Read the model definition and answer for the solid it produces. Units are mm, in the model's axes. A direction names the side the tool comes from. Give positions to 0.01 mm unless a question says otherwise; leave off trailing zeros. Loops run counter-clockwise (first coordinate to the right, second up) from the corner with the lowest first, then second, coordinate; pieces in that order, holes last. Notation, with made-up numbers: (67.25, 82) - (73.25, 82) arc R35 ccw to (73.25, 119) - close; hole circle Ø11 at (-22, 11). An arc over 180 degrees is marked (long way). Put each result on its own line as item: value. Start each with the question number.
1. A cutting plane is placed at A-A, the plane y = 29.5. Determine the outline of the cut face in (x, z), plus the area to 3 significant figures.
2. A cutting plane is placed at D-D, the plane z = 25. Determine the outline of the cut face in (x, y), plus the area to 3 significant figures.
3. For faces 1 (the flat face through (48.877, 46, 20)), 2 (the flat face through (-41.094, 22, 18)), determine the directions among +Z, -Z, +X, -X, +Y, -Y from which every point of the face is accessible in a straight line to the end or side of a thin tool.
4. Consider L1, parallel to X at y = 31, z = 15; L2, parallel to Y at x = 22, z = 8.5; L3, parallel to X at y = 91.5, z = 5. Determine where each line is inside the solid, lowest interval first. Write a range as from..to.
5. A cutting plane is placed at B-B, the plane z = 12. Determine the outline of the cut face in (x, y).
6. A cutting plane is placed at C-C, the plane x = -28. Determine the outline of the cut face in (y, z).
7. Given pin 1 Ø1.5 at (x, y) = (36, -1.5) entering from +Z; pin 2 Ø1.5 at (y, z) = (56.5, 32.5) entering from -X; pin 3 Ø12 at (x, z) = (16.5, 12.5) entering from +Y, each flat-ended and moving along its own axis, determine where each tip first touches the part or whether it passes through.
```python
from build123d import *

# Parameters (mm, degrees)
F0_W     = 11.016868
F0_H     = 24.481927
F0_W_2   = 8.267472
F0_H_2   = 10.750423
F0_W_3   = 4.593041
F0_W_4   = 12.248872
F0_W_5   = 4.59304
F1_DEPTH = 1.836145
F3_DEPTH = 44.06747
F5_DEPTH = 50.8


with BuildPart() as f1:
    # F0 (on Front) → F1 (new body)
    with BuildSketch(Plane.XZ):
        Polygon((-42.930589, 34.886747), (-42.930589, 0), (48.876639, 0), (48.876639, 38.559036), align=None)
        with Locations((-9.046323, 14.077108)):
            Rectangle(F0_W, F0_H, mode=Mode.SUBTRACT)
        with Locations((-28.720862, 20.94286)):
            Rectangle(F0_W_2, F0_H_2, mode=Mode.SUBTRACT)
        with Locations((15.188605, 20.94286)):
            Rectangle(F0_W_3, F0_H_2, mode=Mode.SUBTRACT)
        with Locations((25.274628, 20.94286)):
            Rectangle(F0_W_4, F0_H_2, mode=Mode.SUBTRACT)
        with Locations((35.360651, 20.94286)):
            Rectangle(F0_W_5, F0_H_2, mode=Mode.SUBTRACT)
    extrude(amount=F1_DEPTH)

    # F2 (on face) → F3 (join)
    with BuildSketch(Plane(origin=(0, 0, 0), x_dir=(-1, 0, 0), z_dir=(0, 1, 0))):
        Polygon((42.930589, 0), (42.930589, 34.886747), (41.094445, 34.960193), (41.094445, 0), align=None)
        Polygon((-47.047839, 38.485884), (-48.876639, 38.559036), (-48.876639, 0), (-47.047839, 0), align=None)
    extrude(amount=F3_DEPTH)

    # F4 (on face) → F5 (join)
    with BuildSketch(Plane(origin=(0, 44.06747, 0), x_dir=(-1, 0, 0), z_dir=(0, 1, 0))):
        Polygon((-47.047839, 38.485884), (-48.876639, 38.559036), (-48.876639, 0), (-47.047839, 0), align=None)
    extrude(amount=F5_DEPTH)


solid = f1.part
```
Return value:
1. outline: (-42.93, 0) - (-41.09, 0) - (-41.09, 34.96) - (-42.93, 34.89) - close; (47.05, 0) - (48.88, 0) - (48.88, 38.56) - (47.05, 38.49) - close
1. area: 135 mm2
2. outline: (-42.93, -1.84) - (-32.85, -1.84) - (-32.85, 0) - (-41.09, 0) - (-41.09, 44.07) - (-42.93, 44.07) - close; (-24.59, -1.84) - (-14.55, -1.84) - (-14.55, 0) - (-24.59, 0) - close; (-3.54, -1.84) - (12.89, -1.84) - (12.89, 0) - (-3.54, 0) - close; (17.49, -1.84) - (19.15, -1.84) - (19.15, 0) - (17.49, 0) - close; (31.4, -1.84) - (33.06, -1.84) - (33.06, 0) - (31.4, 0) - close; (37.66, -1.84) - (48.88, -1.84) - (48.88, 94.87) - (47.05, 94.87) - (47.05, 0) - (37.66, 0) - close
2. area: 348 mm2
3. face 1: +Z, -Z, +X, +Y, -Y
3. face 2: +Z, -Z, +Y
4. L1: x = -42.93..-41.09, 47.05..48.88
4. L2: y = -1.84..0
4. L3: x = 47.05..48.88
5. outline: (-42.93, -1.84) - (-14.55, -1.84) - (-14.55, 0) - (-41.09, 0) - (-41.09, 44.07) - (-42.93, 44.07) - close; (-3.54, -1.84) - (48.88, -1.84) - (48.88, 94.87) - (47.05, 94.87) - (47.05, 0) - (-3.54, 0) - close
6. outline: (-1.84, 0) - (0, 0) - (0, 15.57) - (-1.84, 15.57) - close; (-1.84, 26.32) - (0, 26.32) - (0, 35.48) - (-1.84, 35.48) - close
7. pin 1: stops at z = 38.07
7. pin 2: stops at x = 47.05
7. pin 3: stops at y = 0
